Build history of the part. All positions in model axes, mm. Round coordinates to 2 decimals unless told otherwise and drop trailing zeros. Write each loop counter-clockwise with the first axis right and the second up, starting at its lowest first coordinate (ties: lowest second). Pieces come first, ordered by that corner, then holes.
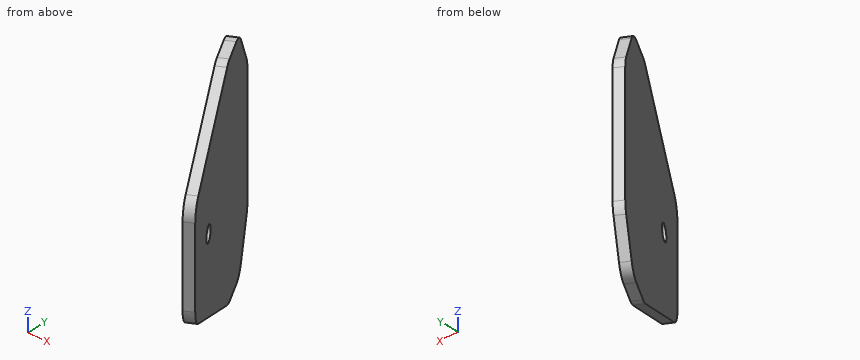
from build123d import *

# Parameters (mm, degrees)
BOSS_EXTRUDE1_DEPTH = 3.175
FILLET1_R           = 6.35
SKETCH2_R           = 2.5
CUT_EXTRUDE1_DEPTH  = 12.192


with BuildPart() as part:
    # Sketch1 → Boss-Extrude1 (new body)
    with BuildSketch(Plane(origin=(460.696994896, 265.983534018, 0), x_dir=(0, 0, -1), z_dir=(0.8660254037844387, 0.49999999999999983, 1.3508489681243032e-15))):
        Polygon((-748.209864924, 226.045570747), (-705.029864924, 226.045570747), (-690.886483256, 216.780668208), (-690.886483256, 204.080668208), (-709.514191369, 165.980668208), (-743.725538479, 165.980668208), (-762.353246592, 204.080668208), (-762.353246592, 216.780668208), align=None)
    extrude(amount=BOSS_EXTRUDE1_DEPTH)

    # Fillet1
    fillet1_edges = [part.edges().sort_by_distance(p)[0] for p in [
        (349.04902485, 462.538490698, 748.209864924),
        (349.04902485, 462.538490698, 705.029864924),
        (353.68147612, 454.514849736, 690.886483256),
        (360.03147612, 443.516327108, 690.886483256),
        (379.08147612, 410.520759223, 709.514191369),
        (379.08147612, 410.520759223, 743.725538479),
        (360.03147612, 443.516327108, 762.353246592),
        (353.68147612, 454.514849736, 762.353246592),
    ]]
    fillet(fillet1_edges, radius=FILLET1_R)

    # Sketch2 → Cut-Extrude1 (cut)
    with BuildSketch(Plane(origin=(463.446625553, 267.571034018, 0), x_dir=(0, 0, -1), z_dir=(0.8660254037844395, 0.4999999999999987, 3.3569404763321265e-15))):
        with Locations(Location((-726.619864924, 181.220668208, 0), (0, 0, 90))):
            Circle(SKETCH2_R)
    extrude(amount=-CUT_EXTRUDE1_DEPTH, mode=Mode.SUBTRACT)


solid = part.part
1) Wall check: L1, parallel to X at y = 461.5, z = 735; L2, parallel to Y at x = 376, z = 736; L3, parallel to X at y = 459, z = 725. Give the ranges that are in metal, low to high.
Results:
L1: x = 347.82 to 351.48
L2: y = 412.68 to 419.03
L3: x = 349.26 to 352.93
2) Slice it at A-A (x = 366.5). Write the cut outline in (y, z).
Results:
outline: (429.14, 698.56) - (435.49, 695.87) - (435.49, 757.37) - (429.14, 754.68) - close
3) Slice it at B-B (z = 698). Write the cut outline in (x, y), plus the area to 3 significant figures.
Results:
outline: (349.98, 457.76) - (365.93, 430.12) - (368.68, 431.71) - (352.73, 459.34) - close
area: 101 mm2
4) Pin check, flat tips, straight feed: pin 1 Ø8 at (y, z) = (421.5, 721.5) entering from -X; pin 2 Ø6 at (x, y) = (351.5, 455) entering from -Z; pin 3 Ø1.5 at (x, y) = (357, 445) entering from +Z; pin 4 Ø1 at (y, z) = (428.5, 707) entering from -X. Stop position of each tip, or through.
Results:
pin 1: stops at x = 368.6
pin 2: stops at z = 691.19
pin 3: stops at z = 762.35
pin 4: stops at x = 366.58
